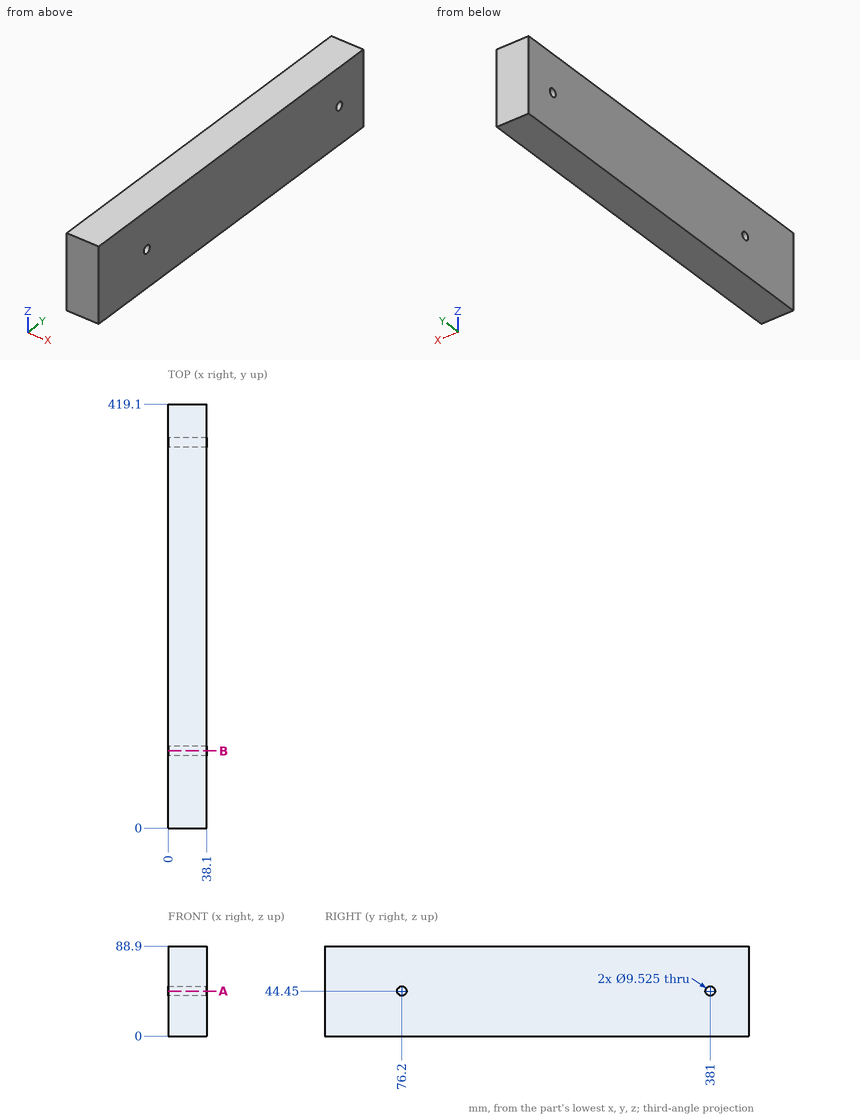
Check sheet for the drawn part. Datum: minimum x, y, z corner. Units: mm. Coordinates: 2 decimals unless noted, no trailing zeros. Write each loop counter-clockwise with the first axis right and the second up, starting at its lowest first coordinate (ties: lowest second). Pieces come first, ordered by that corner, then holes. Notation, with made-up numbers: (2, -9.75) - (31, -9.75) arc R20 ccw to (31, -1.75) - close; hole circle Ø10 at (9.5, -12.5). An arc over 180 degrees is marked (long way). Answer as a JSON object with one key per item and string values.
(1) Thickness scan on line 1 along Y through (x, z) = (21, 44.45); line 2 along Y through (x, z) = (15, 44); line 3 along Z through (x, y) = (28, 76). Record the ranges inside material, lowest first.
Report:
{"line 1": "0 to 71.44, 80.96 to 376.24, 385.76 to 419.1", "line 2": "0 to 71.46, 80.94 to 376.26, 385.74 to 419.1", "line 3": "0 to 39.69, 49.21 to 88.9"}
(2) Cross-section at A-A on z = 44.45. Record the cut outline in (x, y), plus the area to 3 significant figures.
Report:
{"outline": "(0, 0) - (38.1, 0) - (38.1, 71.44) - (0, 71.44) - close; (0, 80.96) - (38.1, 80.96) - (38.1, 376.24) - (0, 376.24) - close; (0, 385.76) - (38.1, 385.76) - (38.1, 419.1) - (0, 419.1) - close", "area": "15,200 mm^2"}
(3) Cross-section at B-B on y = 76.2. Record the cut outline in (x, z).
Report:
{"outline": "(0, 0) - (38.1, 0) - (38.1, 39.69) - (0, 39.69) - close; (0, 49.21) - (38.1, 49.21) - (38.1, 88.9) - (0, 88.9) - close"}
